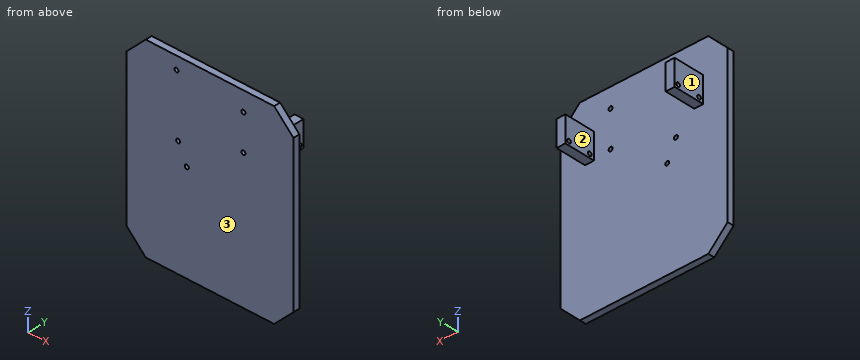
from build123d import *

# Parameters (mm, degrees)
SKETCH1_W           = 130
SKETCH1_H           = 150
BOSS_EXTRUDE1_DEPTH = 2.5
SKETCH4_R           = 1.55
CUT_EXTRUDE2_DEPTH  = 5
SKETCH5_W           = 7
SKETCH5_H           = 20
BOSS_EXTRUDE3_DEPTH = 24
CUT_EXTRUDE3_REACH  = 138.559
SKETCH6_R           = 1.55
CUT_EXTRUDE4_DEPTH  = 5


with BuildPart() as part:
    # Sketch1 → Boss-Extrude1 (new, symmetric)
    with BuildSketch(Plane(origin=(0, 0, 0), x_dir=(1, 0, 0), z_dir=(0, 1, 0))):
        Rectangle(SKETCH1_W, SKETCH1_H)
    extrude(amount=BOSS_EXTRUDE1_DEPTH, both=True)

    # Sketch4 → Cut-Extrude2 (cut)
    with BuildSketch(Plane(origin=(0, 2.5, 0), x_dir=(1, 0, 0), z_dir=(0, 1, 0))):
        with Locations(Location((-24.73, -16.74, 0), (0, 0, 270))):
            Circle(SKETCH4_R)
        with Locations(Location((26.07, -31.98, 0), (0, 0, 270))):
            Circle(SKETCH4_R)
        with Locations(Location((-26, -65, 0), (0, 0, 270))):
            Circle(SKETCH4_R)
        with Locations(Location((26.07, -59.92, 0), (0, 0, 270))):
            Circle(SKETCH4_R)
        with Locations(Location((-18, -2, 0), (0, 0, 270))):
            Circle(SKETCH4_R)
    extrude(amount=-CUT_EXTRUDE2_DEPTH, mode=Mode.SUBTRACT)

    # Sketch5 → Boss-Extrude3 (add)
    with BuildSketch(Plane(origin=(0, 2.5, 0), x_dir=(1, 0, 0), z_dir=(0, 1, 0))):
        with Locations((-42.5, -40)):
            Rectangle(SKETCH5_W, SKETCH5_H)
        with Locations((42.5, -40)):
            Rectangle(SKETCH5_W, SKETCH5_H)
    extrude(amount=BOSS_EXTRUDE3_DEPTH)

    # Cut-Extrude3: up to this face of the body (flat: up to its plane)
    cut_extrude3_end = Plane(part.part.faces().sort_by_distance((46, 14.5, 40))[0])
    # Sketch6 → Cut-Extrude3 (cut, up to the picked face)
    with BuildSketch(Plane.ZY.offset(46), mode=Mode.PRIVATE) as cut_extrude3_sk1:
        with Locations((33, 23.5)):
            Circle(SKETCH6_R)
    cut_extrude3_tool1 = split(extrude(cut_extrude3_sk1.sketch, amount=-CUT_EXTRUDE3_REACH, mode=Mode.PRIVATE), bisect_by=cut_extrude3_end, keep=Keep.BOTH, mode=Mode.PRIVATE)
    # Sketch6 → Cut-Extrude3 (cut, up to the picked face)
    with BuildSketch(Plane.ZY.offset(46), mode=Mode.PRIVATE) as cut_extrude3_sk2:
        with Locations((33, 6)):
            Circle(SKETCH6_R)
    cut_extrude3_tool2 = split(extrude(cut_extrude3_sk2.sketch, amount=-CUT_EXTRUDE3_REACH, mode=Mode.PRIVATE), bisect_by=cut_extrude3_end, keep=Keep.BOTH, mode=Mode.PRIVATE)
    add(cut_extrude3_tool1.solids().sort_by(Axis((-46, 23.5, 33), (1, 0, 0)))[0], mode=Mode.SUBTRACT)
    add(cut_extrude3_tool2.solids().sort_by(Axis((-46, 6, 33), (1, 0, 0)))[0], mode=Mode.SUBTRACT)

    # Sketch7 → Cut-Extrude4 (cut)
    with BuildSketch(Plane(origin=(0, 2.5, 0), x_dir=(1, 0, 0), z_dir=(0, 1, 0))):
        Polygon((-65, -75), (-65, -60), (-50, -75), align=None)
        Polygon((65, -75), (65, -60), (50, -75), align=None)
        Polygon((-65, 75), (-65, 60), (-50, 75), align=None)
        Polygon((65, 75), (65, 60), (50, 75), align=None)
    extrude(amount=-CUT_EXTRUDE4_DEPTH, mode=Mode.SUBTRACT)


solid = part.part
Input: part model. Units: mm. Frame: model coordinates. Face numbers are marked on the shaded views. Coordinates: 2 decimals unless noted, no trailing zeros. Order: outer loops, then holes, each group sorted by start corner. A loop starts at its lowest first (then second) coordinate and runs counter-clockwise, first axis right, second up. Notation, with made-up numbers: M 13,47 L 44,47 A21 cw 44,60 Z; hole C 54.5,81 d9. An arc over 180 degrees is marked long. Answer in a Markdown table with one row per item.
(1) Section query C-C, the plane z = 13. Output: boundary loops of the cut face in (x, y), plus the area to 3 significant figures.
Numbers:
| item | result |
|---|---|
| outline | M -65,-2.5 L 65,-2.5 L 65,2.5 L -65,2.5 Z |
| area | 650 mm^2 |
(2) Material intervals for line 1 (X direction, y = 1.4, z = 65); line 2 (X direction, y = 0.35, z = 59.92); line 3 (Y direction, x = -53, z = -23.5), sorted ascending. Write a range as [from, to].
Numbers:
| item | result |
|---|---|
| line 1 | x = [-60, -27.55], [-24.45, 60] |
| line 2 | x = [-65, 24.52], [27.62, 65] |
| line 3 | y = [-2.5, 2.5] |
(3) Section query B-B, the plane x = 55.5. Output: boundary loops of the cut face in (y, z).
Numbers:
| item | result |
|---|---|
| outline | M -2.5,-69.5 L 2.5,-69.5 L 2.5,69.5 L -2.5,69.5 Z |
(4) Section query A-A, the plane y = 10.75. Output: boundary loops of the cut face in (x, z).
Numbers:
| item | result |
|---|---|
| outline | M -46,30 L -39,30 L -39,50 L -46,50 Z; M 39,30 L 46,30 L 46,50 L 39,50 Z |
(5) Draft query along X for the marked faces 1, 2 and 3. Return one class per face: pulls with the +X half, pulls with the -X half, needs draft (parallel to the pull), parting line crosses it, or undercut.
Numbers:
| item | result |
|---|---|
| face 1 | pulls with the -X half |
| face 2 | undercut |
| face 3 | needs draft |
(6) Contact query for flat-ended pins moving along their axis: pin 1 Ø3.5 at (x, y) = (43, 11) entering from +Z; pin 2 Ø10 at (x, y) = (-19.5, 3.5) entering from +Z; pin 3 Ø6 at (y, z) = (15, 44) entering from +X; pin 4 Ø7.5 at (x, y) = (43.5, 9.5) entering from -Z. Output: stop coordinate, or through.
Numbers:
| item | result |
|---|---|
| pin 1 | stops at z = 50 |
| pin 2 | stops at z = 75 |
| pin 3 | stops at x = 46 |
| pin 4 | stops at z = 30 |
